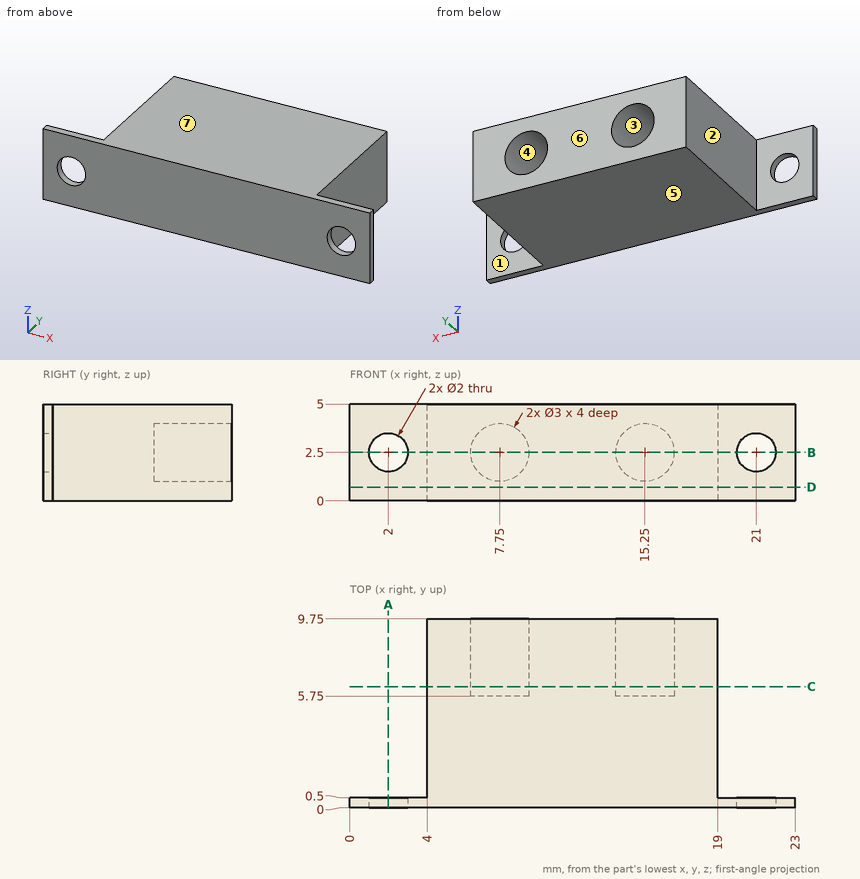
Here's the drawing with two shaded views (mm, measured from the low corner). I have some questions. A direction names the side the tool comes from. Coordinates: 2 decimals unless noted, no trailing zeros. Loops run counter-clockwise (first coordinate to the right, second up) from the corner with the lowest first, then second, coordinate; pieces in that order, holes last. Notation, with made-up numbers: (-17.5, 83) -> (6.5, 83) arc R19 ccw to (6.5, 89) -> close; hole circle Ø9 at (25, 49). An arc over 180 degrees is marked (long way). Put each result on its own line as item: value. Start each with the question number.
Q1. I want a section at D-D (z = 0.7). Write out the boundary of the cut face in (x, y), plus the area to 3 significant figures.
Q2. I want a section at B-B (z = 2.5). Write out the boundary of the cut face in (x, y), plus the area to 3 significant figures.
Q3. For the marked faces 1, 2 and 3, which set-ups out of +Z, -Z, +X, -X, +Y, -Y let a thin tool reach every point of the face, with its end or its side?
Q4. I'm going to push flat-ended pins straight in: P1, Ø2.5, axis at y = 6, z = 3, coming from the +X side; P2, Ø2.5, axis at x = 15.25, z = 2.5, coming from the +Y side; P3, Ø2.5, axis at x = 21, z = 2.5, coming from the +Y side. Where does each tip first touch, or does it pass through?
Q5. I want a section at C-C (y = 6.25). Write out the boundary of the cut face in (x, z).
Q6. I want a section at A-A (x = 2). Write out the boundary of the cut face in (y, z).
Q7. Thinking about a two-plate mould opening in Z: for the marked faces 4, 5, 6 and 7, which applies, pulls with the +Z half, pulls with the -Z half, needs draft (parallel to the pull), parting line crosses it, or undercut?
Q8. If I drill on line 1 (X direction, y = 7.8, z = 2.5); line 2 (X direction, y = 0.45, z = 2.5); line 3 (Z direction, x = 15.25, y = 6.8), over which ranges is the centre line in solid material (lowest first)? Write a range as [from, to].
Taken from the geometry:
1. outline: (0, 0) -> (23, 0) -> (23, 0.5) -> (19, 0.5) -> (19, 9.75) -> (4, 9.75) -> (4, 0.5) -> (0, 0.5) -> close
1. area: 150 mm2
2. outline: (0, 0) -> (1, 0) -> (1, 0.5) -> (0, 0.5) -> close; (3, 0) -> (20, 0) -> (20, 0.5) -> (19, 0.5) -> (19, 9.75) -> (16.75, 9.75) -> (16.75, 5.75) -> (13.75, 5.75) -> (13.75, 9.75) -> (9.25, 9.75) -> (9.25, 5.75) -> (6.25, 5.75) -> (6.25, 9.75) -> (4, 9.75) -> (4, 0.5) -> (3, 0.5) -> close; (22, 0) -> (23, 0) -> (23, 0.5) -> (22, 0.5) -> close
2. area: 124 mm2
3. face 1: +Z, -Z, +X, +Y
3. face 2: +Z, -Z, -X, +Y
3. face 3: +Y
4. P1: stops at x = 19
4. P2: stops at y = 5.75
4. P3: stops at y = 0.5
5. outline: (4, 0) -> (19, 0) -> (19, 5) -> (4, 5) -> close; hole circle Ø3 at (7.75, 2.5); hole circle Ø3 at (15.25, 2.5)
6. outline: (0, 0) -> (0.5, 0) -> (0.5, 1.5) -> (0, 1.5) -> close; (0, 3.5) -> (0.5, 3.5) -> (0.5, 5) -> (0, 5) -> close
7. face 4: undercut
7. face 5: pulls with the -Z half
7. face 6: needs draft
7. face 7: pulls with the +Z half
8. line 1: x = [4, 6.25], [9.25, 13.75], [16.75, 19]
8. line 2: x = [0, 1], [3, 20], [22, 23]
8. line 3: z = [0, 1], [4, 5]
